Here's how the part is built. I have some questions about the finished solid (model axes, mm). Round coordinates to 2 decimals unless told otherwise and drop trailing zeros. Loops run counter-clockwise (first coordinate to the right, second up) from the corner with the lowest first, then second, coordinate; pieces in that order, holes last. Notation, with made-up numbers: M 38.5,22.5 L 58.5,22.5 A8 ccw 58.5,26.5 Z; hole C 82,-16 d1. An arc over 180 degrees is marked long. Answer as CSV lines item,"result".
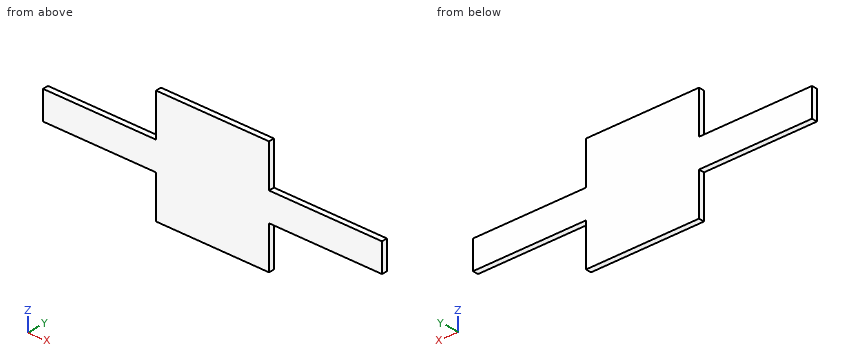
```python
from build123d import *

# Parameters (mm, degrees)
CROQUIS1_W                   = 10
CROQUIS1_H                   = 10
SALIENTE_EXTRUIR1_DEPTH      = 0.5
SALIENTE_EXTRUIR2_DEPTH      = 10
SALIENTE_EXTRUIR2_DEPTH_BACK = 20
CROQUIS2_W                   = 2.5
CROQUIS2_H                   = 0.5


with BuildPart() as part:
    # Croquis1 → Saliente-Extruir1 (new body)
    with BuildSketch(Plane(origin=(0, 0, 0), x_dir=(1, 0, 0), z_dir=(0, 1, 0))):
        with Locations((5, 5)):
            Rectangle(CROQUIS1_W, CROQUIS1_H)
    extrude(amount=SALIENTE_EXTRUIR1_DEPTH)

    # Croquis2 → Saliente-Extruir2 (add, two sides: drawn at the far end of the back side and taken through both)
    with BuildSketch(Plane(origin=(10, 0, 0), x_dir=(0, 0, -1), z_dir=(1, 0, 0)).offset(-SALIENTE_EXTRUIR2_DEPTH_BACK)):
        with Locations((5, 0.25)):
            Rectangle(CROQUIS2_W, CROQUIS2_H)
    extrude(amount=SALIENTE_EXTRUIR2_DEPTH + SALIENTE_EXTRUIR2_DEPTH_BACK)


solid = part.part
```
1. I want a section at C-C, the plane x = -2.75. Please give me the cut outline in (y, z), and give its area (3 significant figures).
Evaluation:
outline,"M 0,-6.25 L 0.5,-6.25 L 0.5,-3.75 L 0,-3.75 Z"
area,"1.25 mm²"
2. If I drill on line 1 (Z direction, x = 13.5, y = 0.1); line 2 (X direction, y = 0.2, z = -2), over which ranges is the centre line in solid material (lowest first)? Write a range as [from, to].
Evaluation:
line 1,"z = [-6.25, -3.75]"
line 2,"x = [0, 10]"
3. I want a section at B-B, the plane z = -2. Please give me the cut outline in (x, y).
Evaluation:
outline,"M 0,0 L 10,0 L 10,0.5 L 0,0.5 Z"
4. I want a section at A-A, the plane y = 0.15. Please give me the cut outline in (x, z), and give its area (3 significant figures).
Evaluation:
outline,"M -10,-6.25 L 0,-6.25 L 0,-10 L 10,-10 L 10,-6.25 L 20,-6.25 L 20,-3.75 L 10,-3.75 L 10,0 L 0,0 L 0,-3.75 L -10,-3.75 Z"
area,"150 mm²"
